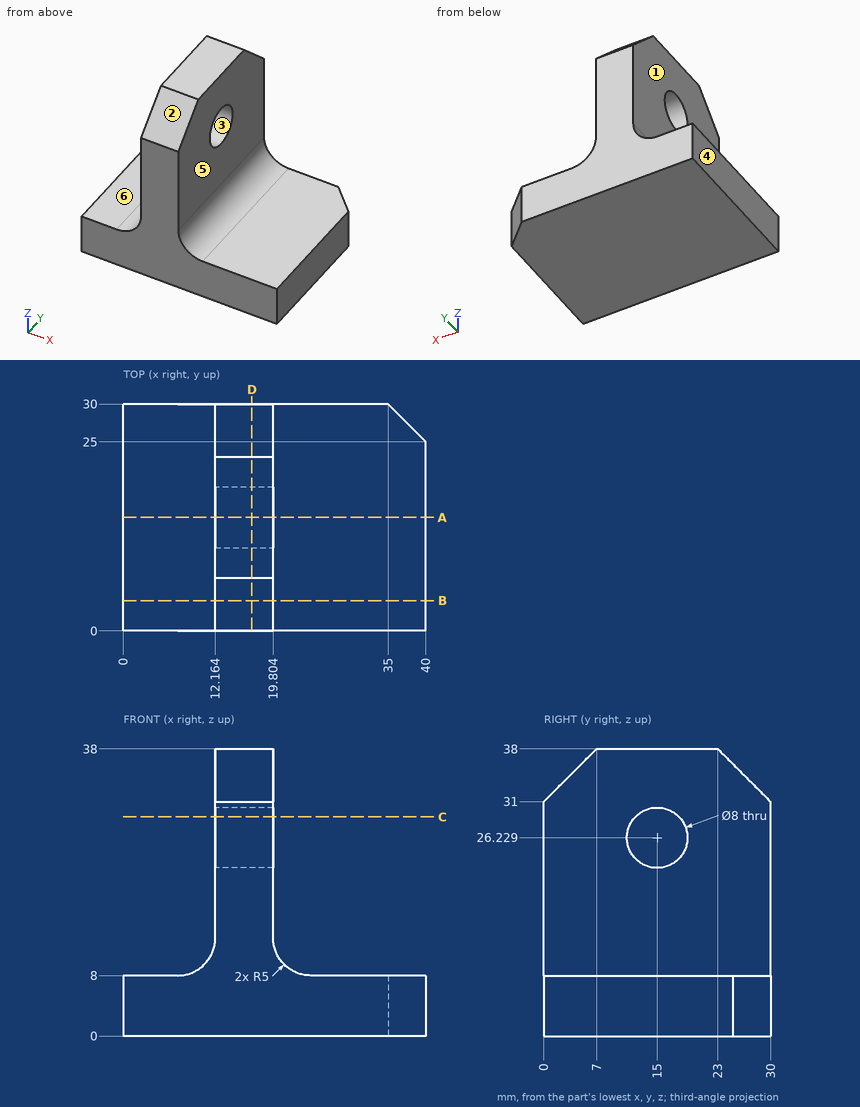
Design review of the part shown in the three views and the two pictorial views. Dimensions are in mm from the part's minimum x, y and z. A direction names the side the tool comes from. Round coordinates to 2 decimals unless told otherwise and drop trailing zeros. Order: outer loops, then holes, each group sorted by start corner. A loop starts at its lowest first (then second) coordinate and runs counter-clockwise, first axis right, second up. Notation, with made-up numbers: (-1.75, 74) - (43.25, 74) arc R25 ccw to (43.25, 106) - close; hole circle Ø5 at (81.5, -29). An arc over 180 degrees is marked (long way). One line per question, with ' | ' between items.
Item 1: Machinability: for the marked faces 4, 5 and 6, which of the approach directions +Z, -Z, +X, -X, +Y, -Y give a long, thin tool a straight path to every point of the face, cutting with its end or side? Answer none if there is none.
Checks:
face 4: +Z, -Z, -X, +Y, -Y | face 5: +Z, +X, +Y, -Y | face 6: +Z, -X, +Y, -Y
Item 2: Take a section at C-C, the plane z = 29. Write out the cut boundary in (x, y) (1 decimal), then the cut area to 3 significant figures.
Checks:
outline: (12.2, 0) - (19.8, 0) - (19.8, 12.1) - (12.2, 12.1) - close; (12.2, 17.9) - (19.8, 17.9) - (19.8, 30) - (12.2, 30) - close | area: 185 mm²
Item 3: Take a section at D-D, the plane x = 17. Write out the cut boundary in (y, z).
Checks:
outline: (0, 0) - (30, 0) - (30, 31) - (23, 38) - (7, 38) - (0, 31) - close; hole circle Ø8 at (15, 26.23)
Item 4: Wall thickness on line 1 (Z direction, x = 17.5, y = 14.75); line 2 (X direction, y = 15, z = 13.5) (1 decimal); line 3 (Z direction, x = 29.5, y = 13): over which ranges is each line inside the solid? List them lowest first. Write a range as [from, to].
Checks:
line 1: [0, 22.24], [30.22, 38] | line 2: [12.2, 19.8] | line 3: [0, 8]
Item 5: Draft analysis for pull direction Z (two halves, no side actions). For the marked faces 1, 2 and 3, state which applies: +Z half, -Z half, draft (parallel to the pull), parting line (faces both ways), or undercut.
Checks:
face 1: draft | face 2: +Z half | face 3: undercut
Item 6: Take a section at A-A, the plane y = 15. Write out the cut boundary in (x, z) (1 decimal), then the cut area to 3 significant figures.
Checks:
outline: (0, 0) - (40, 0) - (40, 8) - (24.8, 8) arc R5 cw to (19.8, 13) - (19.8, 22.2) - (12.2, 22.2) - (12.2, 13) arc R5 cw to (7.2, 8) - (0, 8) - close; (12.2, 30.2) - (19.8, 30.2) - (19.8, 38) - (12.2, 38) - close | area: 499 mm²
Item 7: For P1, Ø3, axis at y = 8, z = 17.5, coming from the +X side; P2, Ø3.5, axis at x = 3.5, y = 18.5, coming from the +Z side; P3, Ø2, axis at y = 5.5, z = 5, coming from the -X side; P4, Ø9, axis at y = 15, z = 26.23, coming from the -X side, all flat-tipped, find the tip position at first contact; note any pin that passes through.
Checks:
P1: x = 19.8 | P2: z = 8 | P3: x = 0 | P4: x = 12.16
Item 8: Take a section at B-B, the plane y = 4. Write out the cut boundary in (x, z) (1 decimal), then the cut area to 3 significant figures.
Checks:
outline: (0, 0) - (40, 0) - (40, 8) - (24.8, 8) arc R5 cw to (19.8, 13) - (19.8, 35) - (12.2, 35) - (12.2, 13) arc R5 cw to (7.2, 8) - (0, 8) - close | area: 537 mm²
